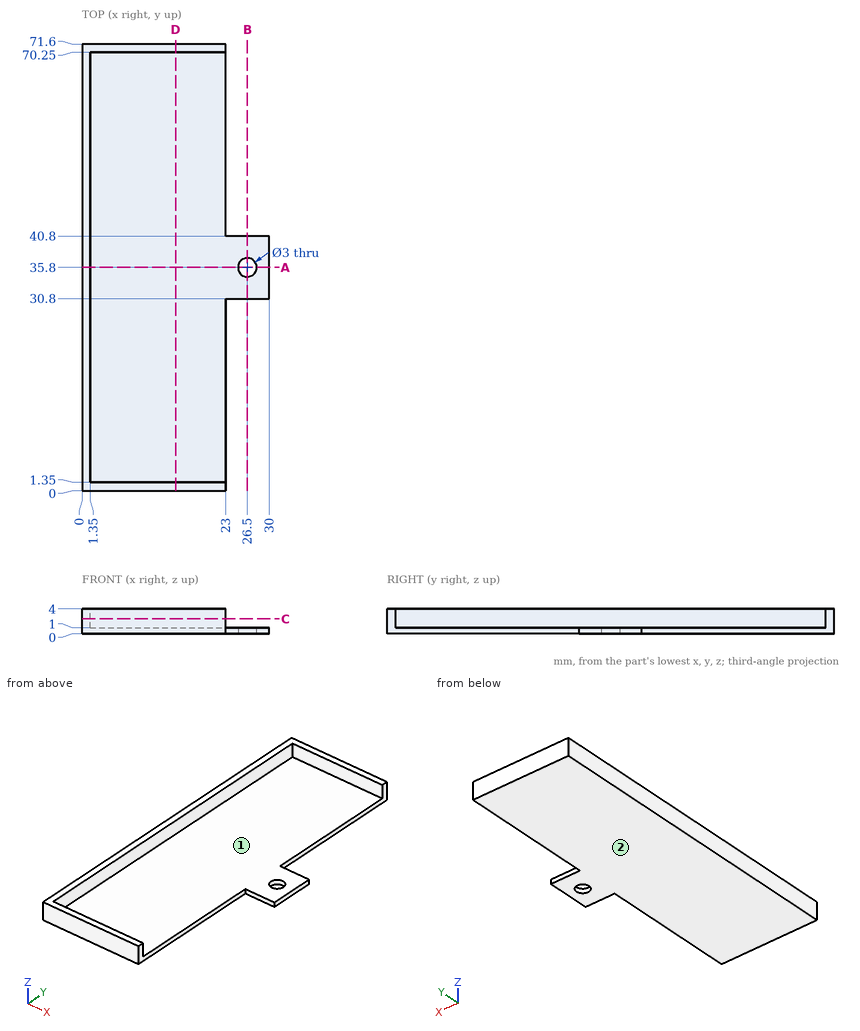
Design review of the part shown in the three views and the two pictorial views. Dimensions are in mm from the part's minimum x, y and z. A direction names the side the tool comes from. Round coordinates to 2 decimals unless told otherwise and drop trailing zeros. Order: outer loops, then holes, each group sorted by start corner. A loop starts at its lowest first (then second) coordinate and runs counter-clockwise, first axis right, second up.
(1) Wall thickness on L1, parallel to Y at x = 15.25, z = 3.85; L2, parallel to Y at x = 26.5, z = 0.75; L3, parallel to Z at x = 14.5, y = 55: over which ranges is each line inside the solid? List them lowest first.
Working result:
L1: y = 0 to 1.35, 70.25 to 71.6
L2: y = 30.8 to 34.3, 37.3 to 40.8
L3: z = 0 to 1
(2) Take a section at D-D, the plane x = 15. State the section outline as (y, z) points.
Working result:
outline: (0, 0) - (71.6, 0) - (71.6, 4) - (70.25, 4) - (70.25, 1) - (1.35, 1) - (1.35, 4) - (0, 4) - close
(3) For P1, Ø1.1, axis at x = 25.5, z = 0.5, coming from the -Y side; P2, Ø1, axis at y = 24.5, z = 0.5, coming from the +X side; P3, Ø2, axis at x = 16.5, y = 64, coming from the -Z side; P4, Ø1.5, axis at x = 26.5, z = 2, coming from the +Y side, all flat-tipped, find the tip position at first contact; note any pin that passes through.
Working result:
P1: stops at y = 30.8
P2: stops at x = 23
P3: stops at z = 0
P4: passes through
(4) Take a section at A-A, the plane y = 35.8. State the section outline as (x, z) points.
Working result:
outline: (0, 0) - (25, 0) - (25, 1) - (1.35, 1) - (1.35, 4) - (0, 4) - close; (28, 0) - (30, 0) - (30, 1) - (28, 1) - close
(5) Take a section at C-C, the plane z = 2.4. State the section outline as (x, y) points.
Working result:
outline: (0, 0) - (23, 0) - (23, 1.35) - (1.35, 1.35) - (1.35, 70.25) - (23, 70.25) - (23, 71.6) - (0, 71.6) - close
(6) Take a section at B-B, the plane x = 26.5. State the section outline as (y, z) points.
Working result:
outline: (30.8, 0) - (34.3, 0) - (34.3, 1) - (30.8, 1) - close; (37.3, 0) - (40.8, 0) - (40.8, 1) - (37.3, 1) - close
(7) Tool access review of the marked faces 1 and 2: name each direction out of +Z, -Z, +X, -X, +Y, -Y from which nothing blocks a thin tool from reaching the whole face with its end or side.
Working result:
face 1: +Z, +X
face 2: -Z, +X, -X, +Y, -Y
